Can you work these out from the model? Positions are in its coordinate system, mm. A direction names the side the tool comes from. Coordinates: 2 decimals unless noted, no trailing zeros. Loops run counter-clockwise (first coordinate to the right, second up) from the corner with the lowest first, then second, coordinate; pieces in that order, holes last.
```python
from build123d import *

# Parameters (mm, degrees)
SKETCH1_R           = 60
BOSS_EXTRUDE1_DEPTH = 60
SKETCH2_R           = 10
CUT_EXTRUDE1_DEPTH  = 20
SKETCH3_R           = 1.5
CUT_EXTRUDE2_DEPTH  = 100


with BuildPart() as part:
    # Sketch1 → Boss-Extrude1 (new body)
    with BuildSketch(Plane(origin=(0, 0, 0), x_dir=(1, 0, 0), z_dir=(0, 1, 0))):
        with Locations(Location((0, 0, 0), (0, 0, 270))):
            Circle(SKETCH1_R)
    extrude(amount=BOSS_EXTRUDE1_DEPTH)

    # Sketch2 → Cut-Extrude1 (cut)
    with BuildSketch(Plane(origin=(0, 0, 0), x_dir=(1, 0, 0), z_dir=(0, 1, 0))):
        with Locations(Location((0, 0, 0), (0, 0, 270))):
            Circle(SKETCH2_R)
    extrude(amount=CUT_EXTRUDE1_DEPTH, mode=Mode.SUBTRACT)

    # Sketch3 → Cut-Extrude2 (cut)
    with BuildSketch(Plane(origin=(0, 0, 0), x_dir=(0, 0, -1), z_dir=(1, 0, 0))):
        with Locations(Location((-15.5, 45.5, 0), (0, 0, 180))):
            Circle(SKETCH3_R)
        with Locations(Location((-15.5, 14.5, 0), (0, 0, 180))):
            Circle(SKETCH3_R)
        with Locations(Location((15.5, 14.5, 0), (0, 0, 180))):
            Circle(SKETCH3_R)
        with Locations(Location((15.5, 45.5, 0), (0, 0, 180))):
            Circle(SKETCH3_R)
    extrude(amount=CUT_EXTRUDE2_DEPTH, mode=Mode.SUBTRACT)


solid = part.part
```
Item 1: Suppose I cut it at D-D, the plane x = 16. Please give me the cut outline in (y, z).
Results are:
outline: (0, -57.83) - (60, -57.83) - (60, 57.83) - (0, 57.83) - close; hole circle Ø3 at (14.5, -15.5); hole circle Ø3 at (14.5, 15.5); hole circle Ø3 at (45.5, -15.5); hole circle Ø3 at (45.5, 15.5)
Item 2: I need wall thicknesses on line 1 along Y through (x, z) = (36.5, 15.5); line 2 along Y through (x, z) = (41, -15); line 3 along Z through (x, y) = (13.5, 14.5). Which ranges of each line are inside material? Lowest first, please.
Results are:
line 1: y = 0 to 13, 16 to 44, 47 to 60
line 2: y = 0 to 13.09, 15.91 to 44.09, 46.91 to 60
line 3: z = -58.46 to -17, -14 to 14, 17 to 58.46
Item 3: Suppose I cut it at C-C, the plane x = -5. Please give me the cut outline in (y, z).
Results are:
outline: (0, -59.79) - (60, -59.79) - (60, 59.79) - (0, 59.79) - (0, 8.66) - (20, 8.66) - (20, -8.66) - (0, -8.66) - close
Item 4: Suppose I cut it at B-B, the plane z = 0. Please give me the cut outline in (x, y), plus the area to 3 significant figures.
Results are:
outline: (-60, 0) - (-10, 0) - (-10, 20) - (10, 20) - (10, 0) - (60, 0) - (60, 60) - (-60, 60) - close
area: 6,800 mm2
Item 5: I'm going to push flat-ended pins straight in: P1, Ø2.5, axis at y = 45.5, z = 15.5, coming from the +X side; P2, Ø3, axis at x = -6.5, y = 50.5, coming from the -Z side; P3, Ø2.5, axis at y = 45, z = 16, coming from the +X side. Where does each tip first touch, or does it pass through?
Results are:
P1: stops at x = 0
P2: stops at z = -59.79
P3: stops at x = 58.04
Item 6: We'd pull the mould along Y, two halves only. Please class faces 4 (the face through (0, 45, -16)), 5 (the face through (1, 0, 12)), 6 (the face through (-9.76, 9.86, -2.17)): +Y half, -Y half, draft (parallel to the pull), parting line (faces both ways), or undercut.
Results are:
face 4: undercut
face 5: -Y half
face 6: draft
Item 7: On a 3-axis mill with a long thin cutter (end or side, diameter ignored), from which of +Z, -Z, +X, -X, +Y, -Y can I reach the whole of each face in a straight line? I mean faces 1 (the face through (0, 20, 0)), 2 (the face through (2.64, 29.58, -59.94)), 3 (the face through (28.77, 14.43, 14)). Say none if no direction works.
Results are:
face 1: -Y
face 2: +Y, -Y
face 3: +X
Item 8: Suppose I cut it at A-A, the plane y = 14.5. Please give me the cut outline in (x, z).
Results are:
outline: (0, -17) - (0, -14) - (58.34, -14) arc R60 ccw to (58.34, 14) - (0, 14) - (0, 17) - (57.54, 17) arc R60 ccw (long way) to (57.54, -17) - close; hole circle Ø20 at (0, 0)
